The model under review builds one solid part; all positions refer to its coordinate system, in mm. A direction names the side the tool comes from. Give positions to 0.01 mm unless a question says otherwise; leave off trailing zeros. Loops run counter-clockwise (first coordinate to the right, second up) from the corner with the lowest first, then second, coordinate; pieces in that order, holes last. Notation, with made-up numbers: M -24.5,-40 L 2.5,-40 A21 ccw 2.5,-12 Z; hole C -26.75,45 d6. An arc over 180 degrees is marked long. Write item = value, one per line. Start each with the question number.
1. For pin 1 (1.5 mm diameter, centred on x = 27, z = 17.5, fed in from +Y); pin 2 (10 mm diameter, centred on x = -18.5, y = 9, fed in from +Z), all flat-tipped, find the tip position at first contact; note any pin that passes through.
2. We need section B-B on x = 0. Give the boundary of the cut face in (y, z), then the cut area to 3 significant figures.
3. We need section A-A on y = 8. Give the boundary of the cut face in (x, z).
4. For faces 4 (the face through (41.5, 18, 45)), 5 (the face through (-4, 2, -48.5)), 6 (the face through (45, 18, 41.5)), list the 3-axis set-ups (+Z, -Z, +X, -X, +Y, -Y) from which the entire face can be reached by the end or side of a thin tool; tool diameter is ignored.
5. Wall thickness on line 1 along X through (y, z) = (14, -44); line 2 along Y through (x, z) = (-22.5, -44); line 3 along Z through (x, y) = (0, 1.8): over which ranges is each line inside the solid? List them lowest first. Write a range as from..to.
6. Draft analysis for pull direction Z (two halves, no side actions). For faces 1 (the face through (45, 18, -41.5)), 2 (the face through (-45, 32.6, 45)), 3 (the face through (4, 2, 48.5)), state which applies: pulls with the +Z half, pulls with the -Z half, needs draft (parallel to the pull), parting line crosses it, or undercut.
7. We need section C-C on z = 0. Give the boundary of the cut face in (x, y), then the cut area to 3 significant figures.
Autodesk Inventor part; units mm, degrees
ref_plane "YZ Plane" through (0, 0, 0) normal (1, 0, 0) x (0, 1, 0)
ref_plane "XZ Plane" through (0, 0, 0) normal (0, 1, 0) x (-1, 0, 0)
ref_plane "XY Plane" through (0, 0, 0) normal (0, 0, 1) x (1, 0, 0)
sketch "Esboço1" plane through (0, 0, 0) normal (0, 1, 0) x (-1, 0, 0)
  line L0 (-46.5, 48.5) -> (46.5, 48.5)
  line L1 (48.5, 46.5) -> (48.5, -46.5)
  line L2 (46.5, -48.5) -> (-46.5, -48.5)
  line L3 (-48.5, -46.5) -> (-48.5, 46.5)
  line L4 (-48.5, 48.5) -> (48.5, -48.5) construction
  line L5 (48.5, 48.5) -> (-48.5, -48.5) construction
  arc A0 (48.5, 46.5) -> (46.5, 48.5) centre (46.5, 46.5) ccw
  arc A1 (-46.5, 48.5) -> (-48.5, 46.5) centre (-46.5, 46.5) ccw
  arc A2 (-48.5, -46.5) -> (-46.5, -48.5) centre (-46.5, -46.5) ccw
  arc A3 (46.5, -48.5) -> (48.5, -46.5) centre (46.5, -46.5) ccw
  point P0 (0, 0)
  dimension "d0" = 97
  dimension "d1" = 97
  dimension "d2" = 2
extrude "Extrusão1" add sketch "Esboço1" along normal blind 3
sketch "Esboço2" plane through (0, 3, 0) normal (0, 1, 0) x (1, 0, 0)
  line L0 (-46.5, -48.5) -> (46.5, -48.5)
  arc A0 (46.5, -48.5) -> (48.5, -46.5) centre (46.5, -46.5) ccw
  line L1 (48.5, -46.5) -> (48.5, 46.5)
  arc A1 (48.5, 46.5) -> (46.5, 48.5) centre (46.5, 46.5) ccw
  line L2 (46.5, 48.5) -> (-46.5, 48.5)
  arc A2 (-46.5, 48.5) -> (-48.5, 46.5) centre (-46.5, 46.5) ccw
  line L3 (-48.5, 46.5) -> (-48.5, -46.5)
  arc A3 (-48.5, -46.5) -> (-46.5, -48.5) centre (-46.5, -46.5) ccw
  line L4 (-46.5, -48.5) -> (-41.5, -48.5)
  line L5 (-41.5, -48.5) -> (-41.5, -41.5)
  line L6 (-41.5, -41.5) -> (-48.5, -41.5)
  line L7 (-48.5, -41.5) -> (-48.5, -46.5)
  line L8 (-46.5, 48.5) -> (-41.5, 48.5)
  line L9 (-41.5, 48.5) -> (-41.5, 41.5)
  line L10 (-41.5, 41.5) -> (-48.5, 41.5)
  line L11 (-48.5, 41.5) -> (-48.5, 46.5)
  line L12 (46.5, -48.5) -> (41.5, -48.5)
  line L13 (41.5, -48.5) -> (41.5, -41.5)
  line L14 (41.5, -41.5) -> (48.5, -41.5)
  line L15 (48.5, -41.5) -> (48.5, -46.5)
  line L16 (46.5, 48.5) -> (41.5, 48.5)
  line L17 (41.5, 48.5) -> (41.5, 41.5)
  line L18 (41.5, 41.5) -> (48.5, 41.5)
  line L19 (48.5, 41.5) -> (48.5, 46.5)
  arc A4 (-48.5, -46.5) -> (-46.5, -48.5) centre (-46.5, -46.5) ccw
  arc A5 (-46.5, 48.5) -> (-48.5, 46.5) centre (-46.5, 46.5) ccw
  arc A6 (48.5, 46.5) -> (46.5, 48.5) centre (46.5, 46.5) ccw
  arc A7 (46.5, -48.5) -> (48.5, -46.5) centre (46.5, -46.5) ccw
  point P0 (0, 0)
  point P1 (-48.5, -48.5)
  point P2 (48.5, 48.5)
  dimension "d6" = 7
  dimension "d7" = 7
  dimension "d8" = 7
  dimension "d9" = 7
  dimension "d10" = 7
  dimension "d11" = 7
  dimension "d12" = 7
  dimension "d13" = 7
  dimension "d14" = 2
sketch "Esboço3" plane through (0, 0, 0) normal (0, -1, 0) x (1, 0, 0)
  circle A0 centre (0, 0) radius 32.5
  dimension "d15" = 65
extrude "Extrusão2" cut sketch "Esboço3" against normal blind 3
extrude "Extrusão3" add sketch "Esboço2" along normal blind 29.6 contours A3 L3 L6 L5 L0 | L13 L14 L1 A0 L0 | L3 A2 L2 L9 L10 | L18 L17 L2 A1 L1
properties part number "suporte interno"
Final values:
q1.pin_1 = 3
q1.pin_2 = through
q2.outline = M 0,-48.5 L 3,-48.5 L 3,-32.5 L 0,-32.5 Z; M 0,32.5 L 3,32.5 L 3,48.5 L 0,48.5 Z
q2.area = 96.0 mm²
q3.outline = M -48.5,-46.5 A2 ccw -46.5,-48.5 L -41.5,-48.5 L -41.5,-41.5 L -48.5,-41.5 Z; M -48.5,41.5 L -41.5,41.5 L -41.5,48.5 L -46.5,48.5 A2 ccw -48.5,46.5 Z; M 41.5,-48.5 L 46.5,-48.5 A2 ccw 48.5,-46.5 L 48.5,-41.5 L 41.5,-41.5 Z; M 41.5,41.5 L 48.5,41.5 L 48.5,46.5 A2 ccw 46.5,48.5 L 41.5,48.5 Z
q4.face_4 = +Z, -Z, +Y
q4.face_5 = -Z, +X, -X, +Y, -Y
q4.face_6 = +X, -X, +Y
q5.line_1 = -48.5..-41.5, 41.5..48.5
q5.line_2 = 0..3
q5.line_3 = -48.5..-32.5, 32.5..48.5
q6.face_1 = undercut
q6.face_2 = needs draft
q6.face_3 = pulls with the +Z half
q7.outline = M -48.5,0 L -32.5,0 L -32.5,3 L -48.5,3 Z; M 32.5,0 L 48.5,0 L 48.5,3 L 32.5,3 Z
q7.area = 96.0 mm²
